from build123d import *

# Parameters (mm, degrees)
F1_DEPTH = 76.2
F2_DEPTH = 6.35
F3_W     = 12.7
F3_H     = 25.4
F4_DEPTH = 6.35
F5_W     = 12.7
F5_H     = 6.35
F5_H_2   = 44.45
F6_DEPTH = 6.35
F7_W     = 12.7
F7_H     = 44.45
F7_H_2   = 6.35
F8_DEPTH = 6.35
F9_R     = 6.35
F10_R    = 6.35


with BuildPart() as f1:
    # F0 (on Top) → F1 (new body)
    with BuildSketch(Plane.XY):
        Polygon((-191.3085826457, -6.122033637), (-168.5362336709, 78.8655297446), (-295.5362336709, 78.8655297446), (-272.7638846962, -6.122033637), align=None)
        Polygon((-267.8913583225, 0.227966363), (-287.2607525534, 72.5155297446), (-176.8117147885, 72.5155297446), (-196.1811090194, 0.227966363), align=None, mode=Mode.SUBTRACT)
    extrude(amount=F1_DEPTH)

    # F0 (on Top) → F2 (join)
    with BuildSketch(Plane.XY):
        Polygon((-176.8117147885, 72.5155297446), (-287.2607525534, 72.5155297446), (-267.8913583225, 0.227966363), (-196.1811090194, 0.227966363), align=None)
    extrude(amount=F2_DEPTH)

    # F3 (on face) → F4 (join)
    with BuildSketch(Plane(origin=(0, 78.8655297446, 0), x_dir=(-1, 0, 0), z_dir=(0, 1, 0))):
        with Locations((200.2862336709, 88.9)):
            Rectangle(F3_W, F3_H)
        with Locations((263.7862336709, 88.9)):
            Rectangle(F3_W, F3_H)
    extrude(amount=-F4_DEPTH)

    # F5 (on face) → F6 (join)
    with BuildSketch(Plane.XY.offset(101.6)):
        with Locations((-200.2862336709, 75.6905297446)):
            Rectangle(F5_W, F5_H)
        with Locations((-200.2862336709, 101.0905297446)):
            Rectangle(F5_W, F5_H_2)
    extrude(amount=F6_DEPTH)

    # F7 (on face) → F8 (join)
    with BuildSketch(Plane.XY.offset(101.6)):
        with Locations((-263.7862336709, 101.0905297446)):
            Rectangle(F7_W, F7_H)
        with Locations((-263.7862336709, 75.6905297446)):
            Rectangle(F7_W, F7_H_2)
    extrude(amount=F8_DEPTH)

    # F9
    f9_edges = [f1.edges().sort_by_distance(p)[0] for p in [
        (-200.286234, 72.51553, 107.95),
    ]]
    fillet(f9_edges, radius=F9_R)

    # F10
    f10_edges = [f1.edges().sort_by_distance(p)[0] for p in [
        (-263.786234, 72.51553, 107.95),
    ]]
    fillet(f10_edges, radius=F10_R)


solid = f1.part
Work out the finished part from the listing and answer in its coordinate system (mm). A direction names the side the tool comes from. Give positions to 0.01 mm unless a question says otherwise; leave off trailing zeros. Write each loop counter-clockwise with the first axis right and the second up, starting at its lowest first coordinate (ties: lowest second). Pieces come first, ordered by that corner, then holes.
Q1. A tool of negligible diameter and unlimited length cuts with its end or side. For faces 1 (the face through (-264, 101, 101.6)), 2 (the face through (-232, 76, 76.2)), 3 (the face through (-233, 72.516, 43)), from which of +Z, -Z, +X, -X, +Y, -Y can it reach the whole face along a straight path? Write none if from no direction.
Answer:
face 1: -Z, +X, -X, +Y
face 2: +Z, +Y, -Y
face 3: +Z
Q2. The part is cut by section A-A on y = 99.5. Give the vertices of the cut face in (x, z), and give its area (3 significant figures).
Answer:
outline: (-270.14, 101.6) - (-257.44, 101.6) - (-257.44, 107.95) - (-270.14, 107.95) - close; (-206.64, 101.6) - (-193.94, 101.6) - (-193.94, 107.95) - (-206.64, 107.95) - close
area: 161 mm2
Q3. Given pin 1 (1.5 mm diameter, centred on x = -226, y = 69, fed in from +Z); pin 2 (1.9 mm diameter, centred on x = -231.5, y = 77, fed in from +Z); pin 3 (10 mm diameter, centred on x = -265, y = 98, fed in from -Z); pin 4 (5 mm diameter, centred on y = 62, z = 79.5, fed in from -X), each flat-ended and moving along its own axis, determine where each tip first touches the part or whether it passes through.
Answer:
pin 1: stops at z = 6.35
pin 2: stops at z = 76.2
pin 3: stops at z = 101.6
pin 4: passes through
Q4. For a pull along X with two mould halves and no side action, classify faces 4 (the face through (-180.08, 35.78, 37.57)), 5 (the face through (-200.197, 74.425, 106.139)), 6 (the face through (-277.44, 35.87, 40.79)) as released by +X, released by -X, zero draft, split by the parting line, or undercut.
Answer:
face 4: released by +X
face 5: zero draft
face 6: undercut
Q5. Straight lines are drawn through the part: L1, parallel to Y at x = -215, z = 68.5; L2, parallel to Y at x = -262, z = 82; L3, parallel to Z at x = -195, y = 29. For each, find the intervals that lie inside material, in ascending order.
Answer:
L1: y = -6.12 to 0.23, 72.52 to 78.87
L2: y = 72.52 to 78.87
L3: z = 0 to 6.35
Q6. The part is cut by section D-D on z = 64. Give the vertices of the cut face in (x, y), and give its area (3 significant figures).
Answer:
outline: (-295.54, 78.87) - (-272.76, -6.12) - (-191.31, -6.12) - (-168.54, 78.87) - close; hole (-287.26, 72.52) - (-267.89, 0.23) - (-196.18, 0.23) - (-176.81, 72.52) - close
area: 2,270 mm2
Q7. The part is cut by section C-C on x = -229.5. Give the vertices of the cut face in (y, z), and give its area (3 significant figures).
Answer:
outline: (-6.12, 0) - (78.87, 0) - (78.87, 76.2) - (72.52, 76.2) - (72.52, 6.35) - (0.23, 6.35) - (0.23, 76.2) - (-6.12, 76.2) - close
area: 1,430 mm2
Q8. The part is cut by section B-B on z = 79.5. Give the vertices of the cut face in (x, y), and give its area (3 significant figures).
Answer:
outline: (-270.14, 72.52) - (-257.44, 72.52) - (-257.44, 78.87) - (-270.14, 78.87) - close; (-206.64, 72.52) - (-193.94, 72.52) - (-193.94, 78.87) - (-206.64, 78.87) - close
area: 161 mm2
